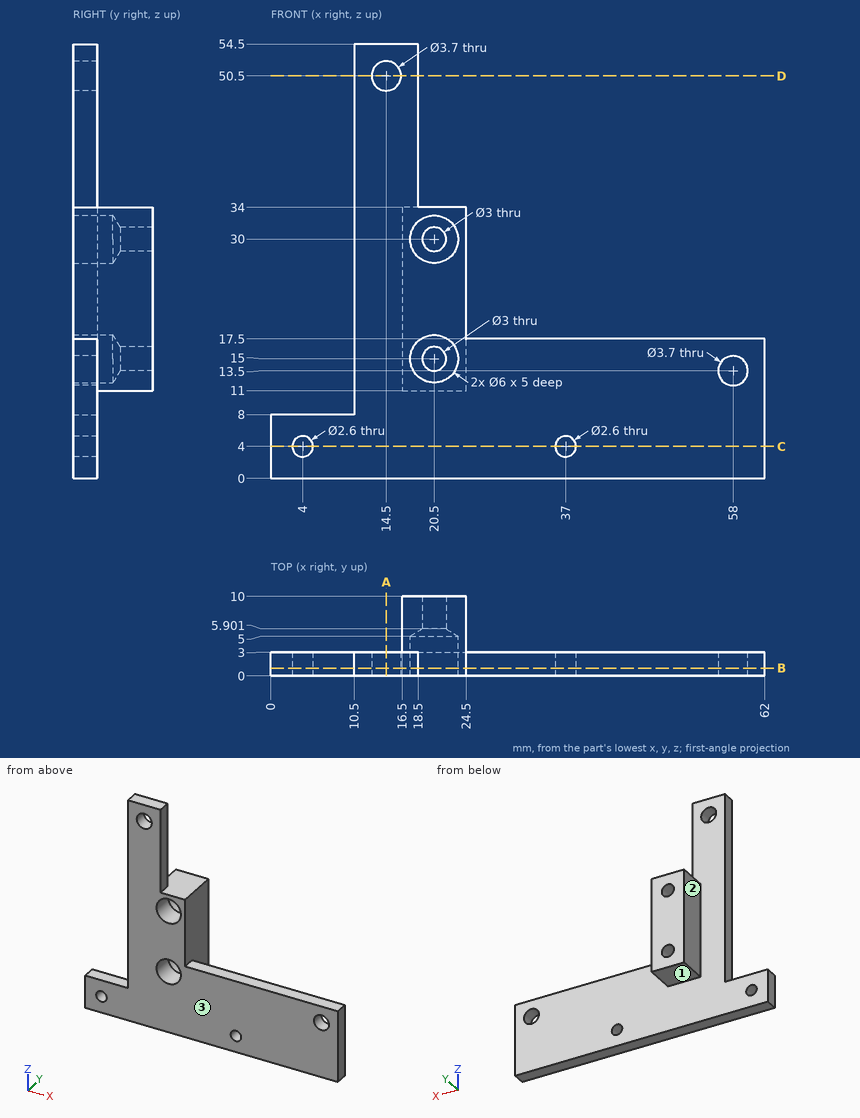
Design review of the part shown in the three views and the two pictorial views. Dimensions are in mm from the part's minimum x, y and z. A direction names the side the tool comes from. Give positions to 0.01 mm unless a question says otherwise; leave off trailing zeros. Loops run counter-clockwise (first coordinate to the right, second up) from the corner with the lowest first, then second, coordinate; pieces in that order, holes last. Notation, with made-up numbers: M 27.25,23.25 L 43.25,23.25 A19 cw 43.25,31.25 Z; hole C 59,-17 d5. An arc over 180 degrees is marked long. Answer as a JSON object with one key per item and string values.
Item 1: We need section D-D (z = 50.5). State the section outline as (x, y) points.
Output values:
{"outline": "M 10.5,0 L 12.65,0 L 12.65,3 L 10.5,3 Z; M 16.35,0 L 18.5,0 L 18.5,3 L 16.35,3 Z"}
Item 2: We need section A-A (x = 14.5). State the section outline as (y, z) points.
Output values:
{"outline": "M 0,0 L 3,0 L 3,48.65 L 0,48.65 Z; M 0,52.35 L 3,52.35 L 3,54.5 L 0,54.5 Z"}
Item 3: We need section B-B (y = 1). State the section outline as (x, z) points, and give its area (3 significant figures).
Output values:
{"outline": "M 0,0 L 62,0 L 62,17.5 L 24.5,17.5 L 24.5,34 L 18.5,34 L 18.5,54.5 L 10.5,54.5 L 10.5,8 L 0,8 Z; hole C 4,4 d2.6; hole C 14.5,50.5 d3.7; hole C 20.5,15 d6; hole C 20.5,30 d6; hole C 37,4 d2.6; hole C 58,13.5 d3.7", "area": "1,290 mm2"}
Item 4: For P1, Ø3, axis at y = 3.5, z = 24, coming from the +X side; P2, Ø3.5, axis at y = 7.5, z = 20.5, coming from the -X side; P3, Ø4, axis at x = 20, y = 6.5, coming from the -Z side; P4, Ø8, axis at x = 20.5, z = 15, coming from the -Y side, all flat-tipped, find the tip position at first contact; note any pin that passes through.
Output values:
{"P1": "stops at x = 24.5", "P2": "stops at x = 16.5", "P3": "stops at z = 11", "P4": "stops at y = 0"}
Item 5: Wall thickness on line 1 along Z through (x, y) = (20.5, 3.85); line 2 along X through (y, z) = (2.3, 30); line 3 along X through (y, z) = (2.8, 15) (1 decimal): over which ranges is each line inside the solid? List them lowest first.
Output values:
{"line 1": "z = 11 to 12, 18 to 27, 33 to 34", "line 2": "x = 10.5 to 17.5, 23.5 to 24.5", "line 3": "x = 10.5 to 17.5, 23.5 to 56.9, 59.1 to 62"}
Item 6: We need section C-C (z = 4). State the section outline as (x, y) points.
Output values:
{"outline": "M 0,0 L 2.7,0 L 2.7,3 L 0,3 Z; M 5.3,0 L 35.7,0 L 35.7,3 L 5.3,3 Z; M 38.3,0 L 62,0 L 62,3 L 38.3,3 Z"}
Item 7: Machinability: for the marked faces 1, 2 and 3, which of the approach directions +Z, -Z, +X, -X, +Y, -Y give a long, thin tool a straight path to every point of the face, cutting with its end or side? Answer none if there is none.
Output values:
{"face 1": "-Z, +X, -X, +Y", "face 2": "+Z, -Z, -X, +Y", "face 3": "+Z, -Z, +X, -X, -Y"}
